Can you work these out from the model? Positions are in its coordinate system, mm. Coordinates: 2 decimals unless noted, no trailing zeros. Order: outer loops, then holes, each group sorted by start corner. A loop starts at its lowest first (then second) coordinate and runs counter-clockwise, first axis right, second up. Notation, with made-up numbers: (40, 3.5) -> (79, 3.5) arc R27 ccw to (79, 39.5) -> close; hole circle Ø9 at (22.25, 16.5). An arc over 180 degrees is marked (long way). Answer in a Markdown table with one row per item.
```python
from build123d import *

# Parameters (mm, degrees)
F0_R     = 35
F1_DEPTH = 1.6


with BuildPart() as f1:
    # F0 (on Top) → F1 (new body)
    with BuildSketch(Plane.XY):
        with BuildLine():
            ThreePointArc((49.638695, -6), (49.909592, -3.005434), (50, 0))
            ThreePointArc((50, 0), (49.909592, 3.005434), (49.638695, 6))
            Line((49.638695, 6), (38, 6))
            Line((38, 6), (38, -6))
            Line((38, -6), (49.638695, -6))
        make_face()
        with BuildLine():
            Line((38, 6), (49.638695, 6))
            ThreePointArc((49.638695, 6), (-50, 0), (49.638695, -6))
            Line((49.638695, -6), (38, -6))
            Line((38, -6), (38, 6))
        make_face()
        Circle(F0_R, mode=Mode.SUBTRACT)
        with BuildLine():
            ThreePointArc((49.638695, 6), (49.909592, 3.005434), (50, 0))
            ThreePointArc((50, 0), (49.909592, -3.005434), (49.638695, -6))
            Line((49.638695, -6), (62, -6))
            Line((62, -6), (62, 6))
            Line((62, 6), (49.638695, 6))
        make_face()
    extrude(amount=F1_DEPTH)


solid = f1.part
```
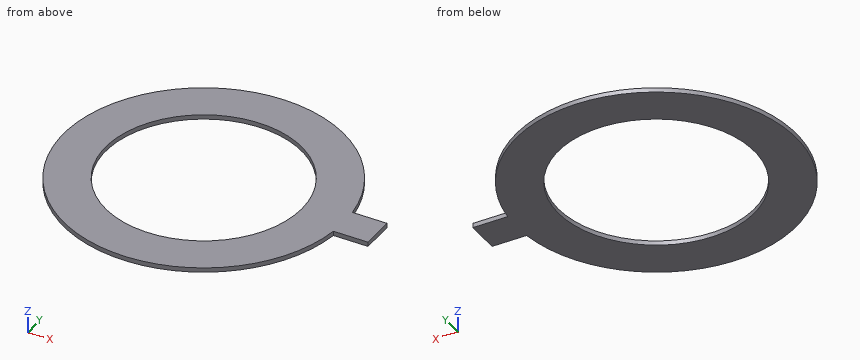
(1) Will this pin go through, and if not, where does the flat tip stop? pin 1 Ø0.5 at (x, z) = (55.5, 0.5) entering from -Y.
Response values:
| item | result |
|---|---|
| pin 1 | y = -6 |
(2) Suppose I cut it at A-A (y = 0). Please give me the cut outline in (x, z), and give its area (3 significant figures).
Response values:
| item | result |
|---|---|
| outline | (-50, 0) -> (-35, 0) -> (-35, 1.6) -> (-50, 1.6) -> close; (35, 0) -> (62, 0) -> (62, 1.6) -> (35, 1.6) -> close |
| area | 67.2 mm2 |
(3) Suppose I cut it at C-C (z = 1). Please give me the cut outline in (x, y).
Response values:
| item | result |
|---|---|
| outline | (49.64, -6) -> (62, -6) -> (62, 6) -> (49.64, 6) arc R50 ccw (long way) to start; hole circle Ø70 at (0, 0) |
(4) I need wall thicknesses on line 1 (Y direction, x = -1, z = 0.65); line 2 (X direction, y = -16, z = 0.95); line 3 (Y direction, x = 10, z = 1.1). Which ranges of each line are inside material? Lowest first, please. Write a range as [from, to].
Response values:
| item | result |
|---|---|
| line 1 | [-49.99, -34.99], [34.99, 49.99] |
| line 2 | [-47.37, -31.13], [31.13, 47.37] |
| line 3 | [-48.99, -33.54], [33.54, 48.99] |
(5) Suppose I cut it at B-B (x = 0). Please give me the cut outline in (y, z).
Response values:
| item | result |
|---|---|
| outline | (-50, 0) -> (-35, 0) -> (-35, 1.6) -> (-50, 1.6) -> close; (35, 0) -> (50, 0) -> (50, 1.6) -> (35, 1.6) -> close |
(6) Suppose I cut it at D-D (x = 46.5). Please give me the cut outline in (y, z), and give its area (3 significant figures).
Response values:
| item | result |
|---|---|
| outline | (-18.38, 0) -> (18.38, 0) -> (18.38, 1.6) -> (-18.38, 1.6) -> close |
| area | 58.8 mm2 |
